```python
from build123d import *

# Parameters (mm, degrees)
CROQUIS1_R              = 4
SALIENTE_EXTRUIR1_DEPTH = 7.5
CORTAR_EXTRUIR1_DEPTH   = 7.5
CORTAR_EXTRUIR2_DEPTH   = 7.5


with BuildPart() as part:
    # Croquis1 → Saliente-Extruir1 (new body, symmetric)
    with BuildSketch(Plane.XY):
        Circle(CROQUIS1_R)
    extrude(amount=SALIENTE_EXTRUIR1_DEPTH, both=True)

    # Croquis2 → Cortar-Extruir1 (cut)
    with BuildSketch(Plane.XY.offset(7.5)):
        with BuildLine():
            Line((-1.532970972, 2.1), (1.532970972, 2.1))
            ThreePointArc((1.532970972, 2.1), (0, -2.6), (-1.532970972, 2.1))
        make_face()
    extrude(amount=-CORTAR_EXTRUIR1_DEPTH, mode=Mode.SUBTRACT)

    # Croquis3 → Cortar-Extruir2 (cut)
    with BuildSketch(Plane(origin=(0, 0, -7.5), x_dir=(-1, 0, 0), z_dir=(0, 0, -1))):
        with BuildLine():
            Line((-2.928736929, 0.65), (2.928736929, 0.65))
            ThreePointArc((2.928736929, 0.65), (0, 3), (-2.928736929, 0.65))
        make_face()
        with BuildLine():
            Line((-2.928736929, -0.65), (2.928736929, -0.65))
            ThreePointArc((2.928736929, -0.65), (0, -3), (-2.928736929, -0.65))
        make_face()
    extrude(amount=-CORTAR_EXTRUIR2_DEPTH, mode=Mode.SUBTRACT)


solid = part.part
```
The model under review builds one solid part; all positions refer to its coordinate system, in mm. A direction names the side the tool comes from. Round coordinates to 2 decimals unless told otherwise and drop trailing zeros. Loops run counter-clockwise (first coordinate to the right, second up) from the corner with the lowest first, then second, coordinate; pieces in that order, holes last. Notation, with made-up numbers: (29.5, 72) - (60.5, 72) arc R13 ccw to (60.5, 87) - close; hole circle Ø4 at (6, 70.5). An arc over 180 degrees is marked (long way). Use a Markdown table: item, result. Add a question column.
Q1. For probe 1 along Y at (x, z) = (-1.25, -6.25); probe 2 along Y at (x, z) = (-2.75, -5.75); probe 3 along Z at (x, y) = (-2.75, 0.75), list the stretches that pass through material, from the lowest coordinate up.
Q2. Add section C-C (z = 5.5). State the section outline as (x, y) points, plus the area to 3 significant figures.
Q3. Add section A-A (x = 0). State the section outline as (y, z) points, plus the area to 3 significant figures.
Q4. Add section B-B (y = -1). State the section outline as (x, z) points.
Q5. Add section D-D (y = 0). State the section outline as (x, z) points.
Q6. The part is to be moulded in two halves that separate along X. For faces 1 (the face through (-0.867, -3.905, 0.105)), 2 (the face through (0, 3, -4)), 3 (the face through (0, 0, -7.5)), say which applies: pulls with the +X half, pulls with the -X half, needs draft (parallel to the pull), parting line crosses it, or undercut.
Q7. Insertion check: pin 1 Ø0.7 at (x, y) = (1.5, 2) entering from -Z; pin 2 Ø1 at (x, z) = (-1.5, 3) entering from +Y; pin 3 Ø1 at (x, z) = (2, 3) entering from +Y. Each pin has a flat end and moves straight along its axis. Give the tip position at first contact, or say it passes through.
Q8. Machinability: for faces 4 (the face through (0, 2.1, 4)), 5 (the face through (0, 0.65, -4)), 6 (the face through (0.1, -2.6, 3.8)), which of the approach directions +Z, -Z, +X, -X, +Y, -Y give a long, thin tool a straight path to every point of the face, cutting with its end or side? Answer none if there is none.
Worked answers:
| question | item | result |
|---|---|---|
| 1 | probe 1 | -3.8 to -2.73, -0.65 to 0.65, 2.73 to 3.8 |
| 1 | probe 2 | -2.9 to -1.2, -0.65 to 0.65, 1.2 to 2.9 |
| 1 | probe 3 | 0 to 7.5 |
| 2 | outline | circle Ø8 at (0, 0); hole (-1.53, 2.1) arc R2.6 ccw (long way) to (1.53, 2.1) - close |
| 2 | area | 30.1 mm² |
| 3 | outline | (-4, -7.5) - (-3, -7.5) - (-3, 0) - (-2.6, 0) - (-2.6, 7.5) - (-4, 7.5) - close; (-0.65, -7.5) - (0.65, -7.5) - (0.65, 0) - (-0.65, 0) - close; (2.1, 0) - (3, 0) - (3, -7.5) - (4, -7.5) - (4, 7.5) - (2.1, 7.5) - close |
| 3 | area | 49.5 mm² |
| 4 | outline | (-3.87, -7.5) - (-2.83, -7.5) - (-2.83, 0) - (-2.4, 0) - (-2.4, 7.5) - (-3.87, 7.5) - close; (2.4, 0) - (2.83, 0) - (2.83, -7.5) - (3.87, -7.5) - (3.87, 7.5) - (2.4, 7.5) - close |
| 5 | outline | (-4, -7.5) - (4, -7.5) - (4, 7.5) - (2.6, 7.5) - (2.6, 0) - (-2.6, 0) - (-2.6, 7.5) - (-4, 7.5) - close |
| 6 | face 1 | parting line crosses it |
| 6 | face 2 | undercut |
| 6 | face 3 | needs draft |
| 7 | pin 1 | z = 0 |
| 7 | pin 2 | y = 3.87 |
| 7 | pin 3 | y = 3.71 |
| 8 | face 4 | +Z, -Z |
| 8 | face 5 | -Z |
| 8 | face 6 | +Z |
